Source: three-view drawing plus pictorial views. Frame: mm from the lowest corner of the part. Coordinates: 2 decimals unless noted, no trailing zeros. Write each loop counter-clockwise with the first axis right and the second up, starting at its lowest first coordinate (ties: lowest second). Pieces come first, ordered by that corner, then holes. Notation, with made-up numbers: (0, 9) - (16, 9) arc R20 cw to (16, 35) - close; hole circle Ø3 at (48.5, 48). An arc over 180 degrees is marked (long way). Answer as a JSON object with one key per item and string values. Group by question number.
Item 1: Line query: line 1 along X through (y, z) = (5.75, 101.6); line 2 along Z through (x, y) = (7.5, 12.5); line 3 along X through (y, z) = (2, 46.5). Output: solid intervals per line, ascending. Write a range as from..to.
Item 2: Section A-A on z = 44.45. Return loops of the section in (x, y).
Item 3: First-contact query: pin 1 Ø3 at (x, y) = (39.5, 4) entering from -Z. Flat tip, straight axial feed; report the tip coordinate or a pass-through.
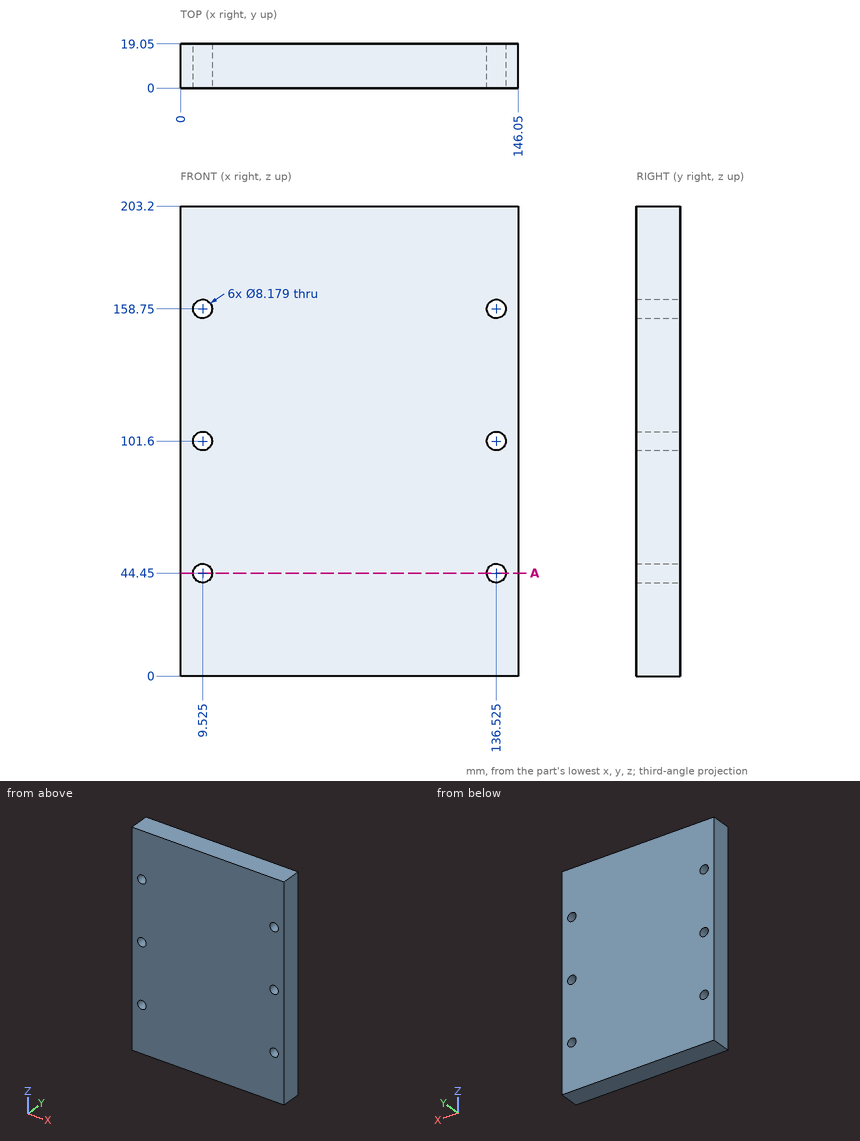
Checks:
{
 "1": {"line 1": "0..5.44, 13.61..132.44, 140.61..146.05", "line 2": "0..40.9, 48..98.05, 105.15..155.2, 162.3..203.2", "line 3": "0..5.99, 13.06..132.99, 140.06..146.05"},
 "2": {"outline": "(0, 0) - (5.44, 0) - (5.44, 19.05) - (0, 19.05) - close; (13.61, 0) - (132.44, 0) - (132.44, 19.05) - (13.61, 19.05) - close; (140.61, 0) - (146.05, 0) - (146.05, 19.05) - (140.61, 19.05) - close"},
 "3": {"pin 1": "z = 0"}
}
